```python
from build123d import *

# Parameters (mm, degrees)
F0_R     = 22.225
F1_DEPTH = 6.35
F2_R     = 14.7955
F3_DEPTH = 6.35
F5_DEPTH = 25.4


with BuildPart() as f1:
    # F0 (on Right) → F1 (new body)
    with BuildSketch(Plane.YZ):
        Circle(F0_R)
    extrude(amount=F1_DEPTH)

    # F2 (on face) → F3 (join)
    with BuildSketch(Plane.YZ.offset(6.35)):
        Circle(F2_R)
    extrude(amount=F3_DEPTH)

    # F4 (on face) → F5 (cut)
    with BuildSketch(Plane(origin=(0, 0, 0), x_dir=(0, -1, 0), z_dir=(-1, 0, 0))):
        with BuildLine():
            ThreePointArc((-17.4797272753, -7.57374639), (-16.4977839421, -9.525), (-15.2989204133, -11.3510146766))
            ThreePointArc((-15.2989204133, -11.3510146766), (-14.5754935306, -10.5624984018), (-14.3133839421, -9.525))
            ThreePointArc((-14.3133839421, -9.525), (-15.3517808132, -7.6653548219), (-17.4797272753, -7.57374639))
        make_face()
        with BuildLine():
            ThreePointArc((-17.4797272753, -7.57374639), (-18.3895298341, -10.6172), (-15.2989204133, -11.3510146766))
            ThreePointArc((-15.2989204133, -11.3510146766), (-16.4977839421, -9.525), (-17.4797272753, -7.57374639))
        make_face()
        with BuildLine():
            ThreePointArc((15.2989204133, -11.3510146766), (16.4977839421, -9.525), (17.4797272753, -7.57374639))
            ThreePointArc((17.4797272753, -7.57374639), (14.6060380501, -8.4328), (15.2989204133, -11.3510146766))
        make_face()
        with BuildLine():
            ThreePointArc((18.6821839421, -9.525), (18.3574291202, -8.3789968711), (17.4797272753, -7.57374639))
            ThreePointArc((17.4797272753, -7.57374639), (16.4977839421, -9.525), (15.2989204133, -11.3510146766))
            ThreePointArc((15.2989204133, -11.3510146766), (17.5352823439, -11.4472904115), (18.6821839421, -9.525))
        make_face()
        with BuildLine():
            ThreePointArc((0, 19.05), (1.0922, 19.0186644946), (2.1808068621, 18.9247610667))
            ThreePointArc((2.1808068621, 18.9247610667), (2.1835015307, 18.9873547666), (2.1844, 19.05))
            ThreePointArc((2.1844, 19.05), (-0.0626452334, 21.2335015307), (-2.1808068621, 18.9247610667))
            ThreePointArc((-2.1808068621, 18.9247610667), (-1.0922, 19.0186644946), (0, 19.05))
        make_face()
        with BuildLine():
            ThreePointArc((0, 16.8656), (1.4996718698, 17.4617343915), (2.1808068621, 18.9247610667))
            ThreePointArc((2.1808068621, 18.9247610667), (1.0922, 19.0186644946), (0, 19.05))
            Line((0, 19.05), (0, 16.8656))
        make_face()
        with BuildLine():
            Line((0, 16.8656), (0, 19.05))
            ThreePointArc((0, 19.05), (-1.0922, 19.0186644946), (-2.1808068621, 18.9247610667))
            ThreePointArc((-2.1808068621, 18.9247610667), (-1.4996718698, 17.4617343915), (0, 16.8656))
        make_face()
    extrude(amount=-F5_DEPTH, mode=Mode.SUBTRACT)


solid = f1.part
```
The listing builds one solid part. Answer for the finished solid, in the listing's coordinates (mm). A direction names the side the tool comes from. Give positions to 0.01 mm unless a question says otherwise; leave off trailing zeros. Order: outer loops, then holes, each group sorted by start corner. A loop starts at its lowest first (then second) coordinate and runs counter-clockwise, first axis right, second up. Notation, with made-up numbers: M 57.25,45 L 105.25,45 A37 cw 105.25,84 Z; hole C -38.75,25.5 d11. An arc over 180 degrees is marked long. Put each result on its own line as item: value. Start each with the question number.
Item 1: Which of the six approach directions +Z, -Z, +X, -X, +Y, -Y give full straight-line access (tool end or side, diameter ignored) to faces 1 (the face through (3.131, 21.199, 6.676)), 2 (the face through (6.35, 5, -15))?
Item 2: Flat-ended cylindrical pins translate along their axes: P1, Ø2, axis at x = 3.5, y = 1, coming from the +Z side (3 decimals); P2, Ø4, axis at y = 16, z = 12.5, coming from the +X side; P3, Ø1.5, axis at x = 4, y = 9, coming from the -Z side. Find the tip coordinate at first contact, or state that the pin passes through.
Item 3: Find the intervals of material crossed by line 1 along Y through (x, z) = (3.75, 20); line 2 along X through (y, z) = (14, 16); line 3 along Z through (x, y) = (5, 14.5), in increasing order.
Item 4: The part is cut by section C-C, the plane y = 8. Determine the outline of the cut face in (x, z).
Item 5: The part is cut by section A-A, the plane x = 5.5. Determine the outline of the cut face in (y, z) (3 decimals).
Answer key:
1. face 1: +X, -X
1. face 2: +X
2. P1: stops at z = 22.225
2. P2: stops at x = 6.35
2. P3: stops at z = -20.64
3. line 1: y = -9.69 to -1.97, 1.97 to 9.69
3. line 2: x = 0 to 6.35
3. line 3: z = -16.84 to -10.41, -8.64 to 16.84
4. outline: M 0,-20.74 L 6.35,-20.74 L 6.35,-12.45 L 12.7,-12.45 L 12.7,12.45 L 6.35,12.45 L 6.35,20.74 L 0,20.74 Z
5. outline: C 0,0 d44.45; hole C -16.498,-9.525 d4.369; hole C 0,19.05 d4.369; hole C 16.498,-9.525 d4.369
